```python
from build123d import *

# Parameters (mm, degrees)
F0_W     = 50
F0_H     = 50
F1_DEPTH = 4
F2_W     = 43.4
F2_H     = 43.4
F3_DEPTH = 3
F4_R     = 3
F4_R_2   = 11
F5_DEPTH = 25
F7_DEPTH = 3
F8_R     = 16
F9_DEPTH = 5
F10_R    = 3


with BuildPart() as f1:
    # F0 (on Front) → F1 (new body)
    with BuildSketch(Plane.XZ):
        Rectangle(F0_W, F0_H)
    extrude(amount=-F1_DEPTH)

    # F2 (on face) → F3 (join)
    with BuildSketch(Plane(origin=(0, 4, 0), x_dir=(-1, 0, 0), z_dir=(0, 1, 0))):
        Rectangle(F2_W, F2_H)
    extrude(amount=F3_DEPTH)

    # F4 (on face) → F5 (cut)
    with BuildSketch(Plane(origin=(0, 7, 0), x_dir=(-1, 0, 0), z_dir=(0, 1, 0))):
        with Locations((-16.5, 16.5)):
            Circle(F4_R)
        with Locations((16.5, 16.5)):
            Circle(F4_R)
        with Locations((16.5, -16.5)):
            Circle(F4_R)
        with Locations((-16.5, -16.5)):
            Circle(F4_R)
        Circle(F4_R_2)
    extrude(amount=-F5_DEPTH, mode=Mode.SUBTRACT)

    # F6 (on face) → F7 (cut)
    with BuildSketch(Plane.XZ):
        Polygon((-19.386751, 11.5), (-13.613249, 11.5), (-10.726497, 16.5), (-13.613249, 21.5), (-19.386751, 21.5), (-22.273503, 16.5), align=None)
        Polygon((19.386751, 21.5), (13.613249, 21.5), (10.726497, 16.5), (13.613249, 11.5), (19.386751, 11.5), (22.273503, 16.5), align=None)
        Polygon((13.613249, -21.5), (19.386751, -21.5), (22.273503, -16.5), (19.386751, -11.5), (13.613249, -11.5), (10.726497, -16.5), align=None)
        Polygon((-19.386751, -21.5), (-13.613249, -21.5), (-10.726497, -16.5), (-13.613249, -11.5), (-19.386751, -11.5), (-22.273503, -16.5), align=None)
    extrude(amount=-F7_DEPTH, mode=Mode.SUBTRACT)

    # F8 (on face) → F9 (cut)
    with BuildSketch(Plane(origin=(0, 7, 0), x_dir=(-1, 0, 0), z_dir=(0, 1, 0))):
        Circle(F8_R)
    extrude(amount=-F9_DEPTH, mode=Mode.SUBTRACT)

    # F10
    f10_edges = [f1.edges().sort_by_distance(p)[0] for p in [
        (21.7, 5.5, 21.7),
        (21.7, 5.5, -21.7),
        (-21.7, 5.5, -21.7),
        (-21.7, 5.5, 21.7),
    ]]
    fillet(f10_edges, radius=F10_R)


solid = f1.part
```
For this review, take the finished solid that the model builds, in its own axes (mm). A direction names the side the tool comes from. Round coordinates to 2 decimals unless told otherwise and drop trailing zeros. Loops run counter-clockwise (first coordinate to the right, second up) from the corner with the lowest first, then second, coordinate; pieces in that order, holes last.
(1) We need section C-C (x = 15). Give the boundary of the cut face in (y, z), plus the area to 3 significant figures.
Returned:
outline: (0, -25) - (4, -25) - (4, -21.7) - (7, -21.7) - (7, -19.1) - (3, -19.1) - (3, -21.5) - (0, -21.5) - close; (0, -11.5) - (3, -11.5) - (3, -13.9) - (7, -13.9) - (7, -5.57) - (2, -5.57) - (2, 5.57) - (7, 5.57) - (7, 13.9) - (3, 13.9) - (3, 11.5) - (0, 11.5) - close; (0, 21.5) - (3, 21.5) - (3, 19.1) - (7, 19.1) - (7, 21.7) - (4, 21.7) - (4, 25) - (0, 25) - close
area: 173 mm2
(2) Clearance check with flat-ended pins moving along their axes: P1, Ø1.5, axis at x = -4, y = 5.5, coming from the -Z side; P2, Ø2.5, axis at x = 4.5, y = 5.5, coming from the +Z side. State where each tip first meets the part, or that it passes through.
Returned:
P1: stops at z = -21.7
P2: stops at z = 21.7
(3) Mouldability with a two-part tool opening along Z and no side actions: class faces 4 (the flat face through (-20.81, 1.479, 19.035)), 5 (the flat face through (-9, 7, -14)), 6 (the flat face through (0, 2, 25)) as released by +Z, released by -Z, zero draft, split by the parting line, or undercut.
Returned:
face 4: undercut
face 5: zero draft
face 6: released by +Z
(4) We need section A-A (z = 0). Give the boundary of the cut face in (x, y).
Returned:
outline: (-25, 0) - (-11, 0) - (-11, 2) - (-16, 2) - (-16, 7) - (-21.7, 7) - (-21.7, 4) - (-25, 4) - close; (11, 0) - (25, 0) - (25, 4) - (21.7, 4) - (21.7, 7) - (16, 7) - (16, 2) - (11, 2) - close
(5) We need section B-B (x = -8). Give the boundary of the cut face in (y, z), plus the area to 3 significant figures.
Returned:
outline: (0, -25) - (4, -25) - (4, -21.7) - (7, -21.7) - (7, -13.86) - (2, -13.86) - (2, -7.55) - (0, -7.55) - close; (0, 7.55) - (2, 7.55) - (2, 13.86) - (7, 13.86) - (7, 21.7) - (4, 21.7) - (4, 25) - (0, 25) - close
area: 161 mm2
(6) We need section D-D (z = -17.5). Give the boundary of the cut face in (x, y), plus the area to 3 significant figures.
Returned:
outline: (-25, 0) - (-21.7, 0) - (-21.7, 3) - (-19.33, 3) - (-19.33, 7) - (-21.7, 7) - (-21.7, 4) - (-25, 4) - close; (-13.67, 3) - (-11.3, 3) - (-11.3, 0) - (11.3, 0) - (11.3, 3) - (13.67, 3) - (13.67, 7) - (-13.67, 7) - close; (19.33, 3) - (21.7, 3) - (21.7, 0) - (25, 0) - (25, 4) - (21.7, 4) - (21.7, 7) - (19.33, 7) - close
area: 223 mm2
(7) Wall thickness on line 1 along Z through (x, y) = (16.5, 4.95); line 2 along X through (y, z) = (5.5, 17.5); line 3 along Z through (x, y) = (0, 0.5): over which ranges is each line inside the solid? List them lowest first.
Returned:
line 1: z = -21.7 to -19.5, -13.5 to 13.5, 19.5 to 21.7
line 2: x = -21.7 to -19.33, -13.67 to 13.67, 19.33 to 21.7
line 3: z = -25 to -11, 11 to 25
(8) Tool access review of faces 1 (the cylindrical face through (-20.8, 5.52, 20.84)), 2 (the flat face through (0, 5, 21.7)), 3 (the flat face through (-14, 3, 19)): name each direction out of +Z, -Z, +X, -X, +Y, -Y from which nothing blocks a thin tool from reaching the whole face with its end or side.
Returned:
face 1: +Z, -X, +Y
face 2: +Z, +X, -X, +Y
face 3: -Y
